Design review of the part built by this model. Coordinates are the model's own, in mm. A direction names the side the tool comes from. Give positions to 0.01 mm unless a question says otherwise; leave off trailing zeros. Loops run counter-clockwise (first coordinate to the right, second up) from the corner with the lowest first, then second, coordinate; pieces in that order, holes last.
from build123d import *

# Parameters (mm, degrees)
F1_DEPTH = 134
F2_DEPTH = 4
F3_W     = 117
F3_H     = 62.9306063323
F4_DEPTH = 1


with BuildPart() as f1:
    # F0 (on Front) → F1 (new body)
    with BuildSketch(Plane.XZ):
        with BuildLine():
            Line((0, 4.45), (0, 0))
            Line((0, 0), (34.9306063323, 0))
            ThreePointArc((34.9306063323, 0), (38.0707858746, 1.5222444749), (38.8209049377, 4.9303637789))
            Line((38.8209049377, 4.9303637789), (14.8801779705, 105.0380623451))
            ThreePointArc((14.8801779705, 105.0380623451), (13.0828693528, 107.5164216279), (10.0595155863, 107.9979971716))
            Line((10.0595155863, 107.9979971716), (-16.2, 101.7180416642))
            Line((-16.2, 101.7180416642), (0, 4.45))
        make_face()
        Polygon((-2.6967180639, 85.6686218319), (13.934308474, 89.6459269865), (26.5407376777, 36.9323808837), (9.9097111398, 32.9550757291), align=None, mode=Mode.SUBTRACT)
        Polygon((26.5407376777, 36.9323808837), (13.934308474, 89.6459269865), (-2.6967180639, 85.6686218319), (9.9097111398, 32.9550757291), align=None)
    extrude(amount=-F1_DEPTH)

    # F0 (on Front) → F2 (cut)
    with BuildSketch(Plane.XZ):
        Polygon((26.5407376777, 36.9323808837), (13.934308474, 89.6459269865), (-2.6967180639, 85.6686218319), (9.9097111398, 32.9550757291), align=None)
    extrude(amount=-F2_DEPTH, mode=Mode.SUBTRACT)

    # F3 (on face) → F4 (join)
    with BuildSketch(Plane(origin=(37.8360580974, 0, 9.0484822786), x_dir=(0, 1, 0), z_dir=(0.9725746513, 0, 0.2325909447))):
        with Locations((67, 49.2310590451)):
            Rectangle(F3_W, F3_H)
    extrude(amount=F4_DEPTH)


solid = f1.part
Q1. Tool access review of faces 4 (the face through (17, 66, 0)), 5 (the face through (27, 125.5, 57)), 6 (the face through (0, 66, 2)), 7 (the face through (20.326, 1.972, 62.92)), 8 (the face through (27, 8.5, 57)): name each direction out of +Z, -Z, +X, -X, +Y, -Y from which nothing blocks a thin tool from reaching the whole face with its end or side.
Results:
face 4: -Z, +X, -X, +Y, -Y
face 5: +Z, +X, +Y
face 6: -Z, -X, +Y, -Y
face 7: -Y
face 8: +Z, +X, -Y
Q2. Insertion check: pin 1 (1.3 mm diameter, centred on y = 66.5, z = 3, fed in from -X); pin 2 (10 mm diameter, centred on y = 91.5, z = 90, fed in from +X); pin 3 (4.5 mm diameter, centred on x = 25, z = 46, fed in from -Y); pin 4 (12 mm diameter, centred on x = -0.5, y = 58, fed in from +Z). Each pin has a flat end and moves straight along its axis. Give the tip position at first contact, or say it passes through.
Results:
pin 1: stops at x = 0
pin 2: stops at x = 20.7
pin 3: stops at y = 0
pin 4: stops at z = 106.91
Q3. Take a section at B-B (z = 52). Give the boundary of the cut face in (x, y), plus the area to 3 significant figures.
Results:
outline: (-7.92, 0) - (5.36, 0) - (5.36, 4) - (22.94, 4) - (22.94, 0) - (27.56, 0) - (27.56, 8.5) - (28.59, 8.5) - (28.59, 125.5) - (27.56, 125.5) - (27.56, 134) - (-7.92, 134) - close
area: 4,800 mm2
Q4. Wall thickness on line 1 (Y direction, x = 17.5, z = 74); line 2 (Z direction, x = 11.5, y = 6); line 3 (Y direction, x = 26, z = 61): over which ranges is each line inside the solid? List them lowest first.
Results:
line 1: y = 4 to 134
line 2: z = 0 to 108.08
line 3: y = 8.5 to 125.5
Q5. Take a section at C-C (x = 7). Give the boundary of the cut face in (y, z), plus the area to 3 significant figures.
Results:
outline: (0, 0) - (134, 0) - (134, 107.27) - (0, 107.27) - (0, 87.99) - (4, 87.99) - (4, 45.12) - (0, 45.12) - close
area: 14,200 mm2
Q6. Take a section at D-D (x = 21.5). Give the boundary of the cut face in (y, z).
Results:
outline: (0, 0) - (134, 0) - (134, 77.36) - (125.5, 77.36) - (125.5, 81.66) - (8.5, 81.66) - (8.5, 77.36) - (0, 77.36) - (0, 58.01) - (4, 58.01) - (4, 35.73) - (0, 35.73) - close
Q7. Take a section at A-A (y = 50). Give the boundary of the cut face in (x, z), plus the area to 3 significant figures.
Results:
outline: (-16.2, 101.72) - (0, 4.45) - (0, 0) - (34.93, 0) arc R4 ccw to (38.82, 4.93) - (33.7, 26.33) - (34.68, 26.56) - (20.04, 87.76) - (19.07, 87.53) - (14.88, 105.04) arc R4 ccw to (10.06, 108) - close
area: 3,790 mm2
Q8. Draft analysis for pull direction X (two halves, no side actions). For faces 1 (the face through (27.255, 66.181, 57.59)), 2 (the face through (-2.9, 66.1, 104.9)), 3 (the face through (12, 4, 62)), state which applies: pulls with the +X half, pulls with the -X half, needs draft (parallel to the pull), parting line crosses it, or undercut.
Results:
face 1: pulls with the +X half
face 2: pulls with the -X half
face 3: undercut
